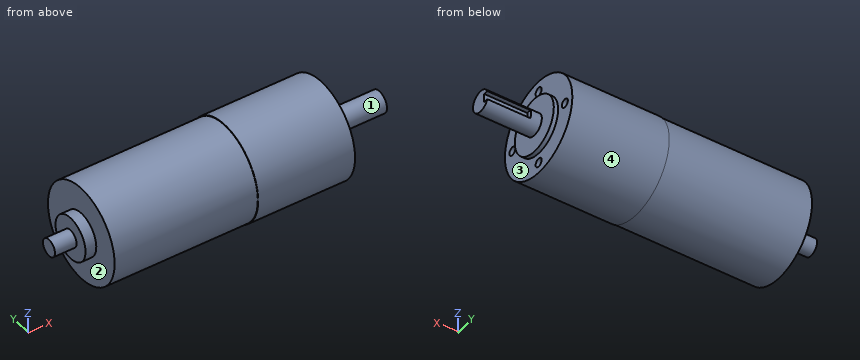
```python
from build123d import *

# Parameters (mm, degrees)
SKETCH1_R           = 5
BOSS_EXTRUDE1_DEPTH = 25
SKETCH2_R           = 13
BOSS_EXTRUDE2_DEPTH = 2
SKETCH3_R           = 22.5
BOSS_EXTRUDE3_DEPTH = 45
SKETCH4_R           = 22.25
BOSS_EXTRUDE4_DEPTH = 66.5
SKETCH5_R           = 10
BOSS_EXTRUDE5_DEPTH = 5
SKETCH6_R           = 4
BOSS_EXTRUDE6_DEPTH = 10
SKETCH7_R           = 2
CUT_EXTRUDE1_DEPTH  = 9
SKETCH8_W           = 4
SKETCH8_H           = 2.5
CUT_EXTRUDE2_DEPTH  = 20


with BuildPart() as part:
    # Sketch1 → Boss-Extrude1 (new body)
    with BuildSketch(Plane(origin=(0, 0, 0), x_dir=(0, 0, -1), z_dir=(1, 0, 0))):
        Circle(SKETCH1_R)
    extrude(amount=-BOSS_EXTRUDE1_DEPTH)

    # Sketch2 → Boss-Extrude2 (add)
    with BuildSketch(Plane.ZY.offset(25)):
        Circle(SKETCH2_R)
    extrude(amount=BOSS_EXTRUDE2_DEPTH)

    # Sketch3 → Boss-Extrude3 (add)
    with BuildSketch(Plane.ZY.offset(27)):
        with Locations(Location((0, 0, 0), (0, 0, 180))):
            Circle(SKETCH3_R)
    extrude(amount=BOSS_EXTRUDE3_DEPTH)

    # Sketch4 → Boss-Extrude4 (add)
    with BuildSketch(Plane.ZY.offset(72)):
        Circle(SKETCH4_R)
    extrude(amount=BOSS_EXTRUDE4_DEPTH)

    # Sketch5 → Boss-Extrude5 (add)
    with BuildSketch(Plane.ZY.offset(138.5)):
        Circle(SKETCH5_R)
    extrude(amount=BOSS_EXTRUDE5_DEPTH)

    # Sketch6 → Boss-Extrude6 (add)
    with BuildSketch(Plane.ZY.offset(143.5)):
        Circle(SKETCH6_R)
    extrude(amount=BOSS_EXTRUDE6_DEPTH)

    # Sketch7 → Cut-Extrude1 (cut)
    with BuildSketch(Plane(origin=(-27, 0, 0), x_dir=(0, 0, -1), z_dir=(1, 0, 0))):
        with Locations((0, 17.5)):
            Circle(SKETCH7_R)
        with Locations((17.5, 0)):
            Circle(SKETCH7_R)
        with Locations((0, -17.5)):
            Circle(SKETCH7_R)
        with Locations((-17.5, 0)):
            Circle(SKETCH7_R)
    extrude(amount=-CUT_EXTRUDE1_DEPTH, mode=Mode.SUBTRACT)

    # Sketch8 → Cut-Extrude2 (cut)
    with BuildSketch(Plane(origin=(0, 0, 0), x_dir=(0, 0, -1), z_dir=(1, 0, 0))):
        with Locations((0, 3.75)):
            Rectangle(SKETCH8_W, SKETCH8_H)
    extrude(amount=-CUT_EXTRUDE2_DEPTH, mode=Mode.SUBTRACT)


solid = part.part
```
Geometry check sheet. Reference: the model listing, model coordinates, mm. Face numbers are marked on the shaded views. A direction names the side the tool comes from. Round coordinates to 2 decimals unless told otherwise and drop trailing zeros. Loops run counter-clockwise (first coordinate to the right, second up) from the corner with the lowest first, then second, coordinate; pieces in that order, holes last. Notation, with made-up numbers: (73, 35) - (108, 35) arc R10 cw to (108, 39) - close; hole circle Ø3 at (16.5, -15). An arc over 180 degrees is marked (long way). Write each question's results on one line, items separated by ' | '. Start each with the question number.
Q1. Thickness scan on line 1 (Y direction, x = -32.5, z = 0); line 2 (X direction, y = -4.5, z = -9); line 3 (X direction, y = 8.5, z = 14.5). Record the ranges inside material, lowest first. Write a range as [from, to].
Q2. Gauge pin test, flat ends, axial feed: P1, Ø3.5, axis at y = 17.5, z = 0, coming from the +X side; P2, Ø1.5, axis at x = -33.5, y = 17, coming from the -Z side; P3, Ø0.6, axis at x = -7, y = 4, coming from the -Z side. Record the tip position at first contact, or that the pin passes through.
Q3. Release check for a two-part mould opening along Y. For the marked faces 3 and 4 record: +Y half, -Y half, draft (parallel to the pull), parting line (faces both ways), or undercut.
Q4. Access from +Z, -Z, +X, -X, +Y, -Y to the whole of each face (thin tool, end or side, straight path). Record for the marked faces 1 and 2.
Q5. Cross-section at C-C on x = -140. Enter the section's corners in (y, z), and give its area (3 significant figures).
Q6. Cross-section at D-D on z = 17. Enter the section's corners in (x, y), and give its area (3 significant figures).
Answers below:
1) line 1: y = [-22.5, -19.5], [-15.5, 15.5], [19.5, 22.5] | line 2: x = [-138.5, -25] | line 3: x = [-138.5, -27]
2) P1: stops at x = -36 | P2: stops at z = -15.56 | P3: stops at z = -3.36
3) face 3: draft | face 4: parting line
4) face 1: +X | face 2: -X
5) outline: circle Ø20 at (0, 0) | area: 314 mm²
6) outline: (-138.5, -14.35) - (-72, -14.35) - (-72, -14.74) - (-27, -14.74) - (-27, -1.94) - (-36, -1.94) - (-36, 1.94) - (-27, 1.94) - (-27, 14.74) - (-72, 14.74) - (-72, 14.35) - (-138.5, 14.35) - close | area: 3,200 mm²
